from build123d import *

# Parameters (mm, degrees)
CUT_EXTRUDE3_DEPTH      = 563.167093213
CUT_EXTRUDE3_DEPTH_BACK = 563.167093213
SKETCH21_R              = 5


with BuildPart() as part:
    # Sweep-Thin3: sweep along a curve in space
    with BuildLine() as sweep_thin3_path:
        Line((0, 0, 0), (430, 0, 0))
        Line((430, 0, 0), (520.097414894, -91.087777242, 127.5))
        Line((520.097414894, -91.087777242, 127.5), (520.097414894, -91.087777242, 157.5))
    # Sketch2 → Sweep-Thin3 (sweep)
    with BuildSketch(Plane(origin=(0, 0, 0), x_dir=(0, 0, -1), z_dir=(1, 0, 0))):
        with BuildLine():
            Line((1.5, 9.5), (-1.5, 9.5))
            ThreePointArc((-1.5, 9.5), (-7.156854249, 7.156854249), (-9.5, 1.5))
            Line((-9.5, 1.5), (-9.5, -1.5))
            ThreePointArc((-9.5, -1.5), (-7.156854249, -7.156854249), (-1.5, -9.5))
            Line((-1.5, -9.5), (1.5, -9.5))
            ThreePointArc((1.5, -9.5), (7.156854249, -7.156854249), (9.5, -1.5))
            Line((9.5, -1.5), (9.5, 1.5))
            ThreePointArc((9.5, 1.5), (7.156854249, 7.156854249), (1.5, 9.5))
        make_face()
        with BuildLine():
            Line((1.5, 6.5), (-1.5, 6.5))
            ThreePointArc((-1.5, 6.5), (-5.035533906, 5.035533906), (-6.5, 1.5))
            Line((-6.5, 1.5), (-6.5, -1.5))
            ThreePointArc((-6.5, -1.5), (-5.035533906, -5.035533906), (-1.5, -6.5))
            Line((-1.5, -6.5), (1.5, -6.5))
            ThreePointArc((1.5, -6.5), (5.035533906, -5.035533906), (6.5, -1.5))
            Line((6.5, -1.5), (6.5, 1.5))
            ThreePointArc((6.5, 1.5), (5.035533906, 5.035533906), (1.5, 6.5))
        make_face(mode=Mode.SUBTRACT)
    sweep(path=sweep_thin3_path.line, transition=Transition.RIGHT)

    # Sketch21 → Cut-Extrude3 (cut, two sides: drawn at the far end of the back side and taken through both)
    with BuildSketch(Plane(origin=(0, 0, 0), x_dir=(1, 0, 0), z_dir=(0, 1, 0)).offset(-CUT_EXTRUDE3_DEPTH_BACK)):
        with Locations(Location((50, 0, 0), (0, 0, 342.542396876))):
            Circle(SKETCH21_R)
    extrude(amount=CUT_EXTRUDE3_DEPTH + CUT_EXTRUDE3_DEPTH_BACK, mode=Mode.SUBTRACT)


solid = part.part
For this review, take the finished solid that the model builds, in its own axes (mm). A direction names the side the tool comes from. Round coordinates to 2 decimals unless told otherwise and drop trailing zeros. Loops run counter-clockwise (first coordinate to the right, second up) from the corner with the lowest first, then second, coordinate; pieces in that order, holes last. Notation, with made-up numbers: (48.25, 65) - (94.25, 65) arc R20 ccw to (94.25, 78) - close; hole circle Ø7 at (-1.75, 88). An arc over 180 degrees is marked (long way). Use one line per item in the form item = value.
1) Mouldability with a two-part tool opening along Z and no side actions: class faces 1 (the face through (477.11, -53.93, 58.29)), 2 (the face through (480.095, -47.524, 60.051)), 3 (the face through (523.349, -100.672, 140.678)) as pulls with the +Z half, pulls with the -Z half, needs draft (parallel to the pull), parting line crosses it, or undercut.
Solutions:
face_1 = pulls with the -Z half
face_2 = undercut
face_3 = needs draft
2) We need section B-B on x = 382. Write out the cut boundary in (y, z).
Solutions:
outline = (-9.5, -1.5) arc R8 ccw to (-1.5, -9.5) - (1.5, -9.5) arc R8 ccw to (9.5, -1.5) - (9.5, 1.5) arc R8 ccw to (1.5, 9.5) - (-1.5, 9.5) arc R8 ccw to (-9.5, 1.5) - close; hole (-6.5, -1.5) arc R5 ccw to (-1.5, -6.5) - (1.5, -6.5) arc R5 ccw to (6.5, -1.5) - (6.5, 1.5) arc R5 ccw to (1.5, 6.5) - (-1.5, 6.5) arc R5 ccw to (-6.5, 1.5) - close
3) Tool access review of faces 4 (the face through (510.5, -94.3, 142.3)), 5 (the face through (473.159, -52.334, 64.135)), 6 (the face through (516.85, -81.5, 143.65)), 7 (the face through (0, -6.5, -4.4)): name each direction out of +Z, -Z, +X, -X, +Y, -Y from which nothing blocks a thin tool from reaching the whole face with its end or side.
Solutions:
face_4 = +Z, -X
face_5 = none
face_6 = +Z, +Y
face_7 = +Z, -Z, -X, +Y, -Y
4) We need section A-A on z = 139. Write out the cut boundary in (x, y).
Solutions:
outline = (510.89, -88.31) arc R8 ccw to (514.62, -98.99) - (517.32, -100.3) arc R8 ccw to (528, -96.57) - (529.31, -93.87) arc R8 ccw to (525.58, -83.18) - (522.88, -81.88) arc R8 ccw to (512.19, -85.61) - close; hole (513.59, -89.61) arc R5 ccw to (515.92, -96.29) - (518.62, -97.59) arc R5 ccw to (525.3, -95.26) - (526.6, -92.56) arc R5 ccw to (524.27, -85.89) - (521.57, -84.58) arc R5 ccw to (514.9, -86.91) - close
5) We need section C-C on x = 50. Write out the cut boundary in (y, z).
Solutions:
outline = (-8.69, -5) arc R8 ccw to (-1.5, -9.5) - (1.5, -9.5) arc R8 ccw to (8.69, -5) - (5.07, -5) arc R5 cw to (1.5, -6.5) - (-1.5, -6.5) arc R5 cw to (-5.07, -5) - close; (-8.69, 5) - (-5.07, 5) arc R5 cw to (-1.5, 6.5) - (1.5, 6.5) arc R5 cw to (5.07, 5) - (8.69, 5) arc R8 ccw to (1.5, 9.5) - (-1.5, 9.5) arc R8 ccw to start
6) Wall thickness on probe 1 along X at (y, z) = (-7.5, 0); probe 2 along X at (y, z) = (-6.65, 0); probe 3 along Y at (x, z) = (305.5, 2): over which ranges is each line inside the solid? List them lowest first.
Solutions:
probe_1 = 0 to 45, 55 to 429.46, 436.35 to 440.95
probe_2 = 0 to 45, 55 to 428.06, 436.94 to 441.23
probe_3 = -9.48 to -6.47, 6.47 to 9.48
7) Clearance check with flat-ended pins moving along their axes: P1, Ø3.5, axis at x = 256, y = 0.5, coming from the +Z side; P2, Ø3.5, axis at x = 30, z = -0.5, coming from the -Y side; P3, Ø4, axis at x = 436, y = -20.5, coming from the +Z side. State where each tip first meets the part, or that it passes through.
Solutions:
P1 = 9.5
P2 = -9.5
P3 = 27.56
